Autodesk Fusion 360 part; units mm, degrees
sketch "Sketch1" plane through (0, 0, 0) normal (1, 0, 0) x (0, 0, -1)
  circle A0 centre (0, 0) radius 4
  line L0 (2, 2) -> (-2, 2)
  line L1 (-2, 2) -> (-2, -2)
  line L2 (-2, -2) -> (2, -2)
  line L3 (2, -2) -> (2, 2)
  line L4 (2, 2) -> (-2, -2) construction
  line L5 (-2, 2) -> (2, -2) construction
  dimension "d1" = 8
  dimension "d2" = 4
  dimension "d3" = 4
extrude "Extrude1" add sketch "Sketch1" along normal blind 2
sketch "Sketch2" plane through (2, 0, 0) normal (1, 0, 0) x (0, 0, -1)
  line L0 (2, 2) -> (2, -2)
  line L1 (2, -2) -> (-2, -2)
  line L2 (-2, -2) -> (-2, 2)
  line L3 (-2, 2) -> (2, 2)
  circle A0 centre (0, 0) radius 4
  circle A1 centre (0, 0) radius 7.5
  dimension "d6" = 15
extrude "Extrude2" add sketch "Sketch2" along normal blind 2 contours L0 L1 L2 L3 | A0 | A1
fillet "Fillet1" radius 1 1 edges at (2, -1.4465, 3.7293)
chamfer "Chamfer1" distance 0.5 angle 45 1 edges at (4, -2.7121, 6.9925)
sketch "Sketch3" plane through (4, 0, 0) normal (1, 0, 0) x (0, 0, -1)
  circle A0 centre (0, 0) radius 7
  line L0 (0, 0) -> (0, 2)
  line L1 (0, -4.8) -> (2, -4.8)
  line L2 (2, -4.8) -> (2, -5.6)
  line L3 (2, -5.6) -> (-2, -5.6)
  line L4 (-2, -5.6) -> (-2, -4.8)
  line L5 (0, -4.8) -> (-2, -4.8)
  line L6 (0, -3) -> (1.5, -3)
  line L7 (0, -3.8) -> (1.5, -3.8)
  line L8 (0, -3) -> (-1.5, -3)
  line L9 (0, -3.8) -> (-1.5, -3.8)
  line L10 (2.5, 2) -> (2.5, 0)
  line L11 (-2.5, 2) -> (-2.5, 0)
  line L12 (-1.7, 2) -> (-2.5, 2) construction
  line L13 (0, 2) -> (2.5, 2) construction
  line L14 (-1.7, 2) -> (-1.7, 0)
  line L15 (1.7, 2) -> (1.7, 0)
  arc A1 (-1.6925, 0.16) -> (1.6925, 0.16) centre (0, 0) ccw
  arc A2 (1.6925, 1.84) -> (-1.6925, 1.84) centre (0, 2) ccw
  arc A3 (-1.6925, 1.84) -> (-1.7, 1.833) centre (0, 0) ccw
  arc A4 (-1.7, 0.167) -> (-1.6925, 0.16) centre (0, 2) ccw
  arc A5 (-2.5, 0) -> (2.5, 0) centre (0, 0) ccw
  arc A6 (1.7, 1.833) -> (1.6925, 1.84) centre (0, 0) ccw
  arc A7 (1.6925, 0.16) -> (1.7, 0.167) centre (0, 2) ccw
  arc A8 (2.5, 2) -> (-2.5, 2) centre (0, 2) ccw
  line L16 (3, -1.5) -> (3.8, -1.5)
  arc A9 (1.5, -3) -> (3, -1.5) centre (1.5, -1.5) ccw
  arc A10 (1.5, -3.8) -> (3.8, -1.5) centre (1.5, -1.5) ccw
  line L17 (-3, -1.5) -> (-3.8, -1.5)
  arc A11 (-3.8, -1.5) -> (-1.5, -3.8) centre (-1.5, -1.5) ccw
  arc A12 (-3, -1.5) -> (-1.5, -3) centre (-1.5, -1.5) ccw
  line L18 (-0.4, -3.8) -> (0.4, -3.8)
  line L19 (0.4, -3.8) -> (0.4, -4.8)
  line L20 (0.4, -4.8) -> (-0.4, -4.8)
  line L21 (-0.4, -4.8) -> (-0.4, -3.8)
  dimension "d12" = 0.8
  dimension "d13" = 0.8
  dimension "d14" = 0.8
  dimension "d15" = 5
  dimension "d16" = 5
  dimension "d17" = 2
  dimension "d18" = 0.8
  dimension "d19" = 3
  dimension "d20" = 1.5
  dimension "d21" = 1.5
  dimension "d24" = 1.5
  dimension "d25" = 0.8
  dimension "d26" = 1.5
  dimension "d27" = 0.8
  dimension "d28" = 0.8
  dimension "d29" = 1.5
  dimension "d30" = 4
  dimension "d31" = 2
  dimension "d32" = 1
  dimension "d33" = 0.8
  dimension "d34" = 0.4
extrude "Extrude3" cut sketch "Sketch3" against normal blind 0.4 contours L1 L5 L7 L9 L18 L19 L20 L21 | L1 L2 L3 L4 L5 L20 | L6 L7 L8 L9 L16 A9 A10 L17 A11 A12 L18 | L10 L11 A5 A8
fillet "Fillet2" radius 0.4 12 edges at (3.8, -5.6, 2) (3.8, -4.8, 2) (3.8, -4.8, 0.4) (3.8, -3.8, 0.4) (3.8, -4.8, -2) (3.8, -5.6, -2) (3.8, -4.8, -0.4) (3.8, -3.8, -0.4) (3.8, -1.5, 3) (3.8, -1.5, 3.8) (3.8, -1.5, -3.8) (3.8, -1.5, -3)
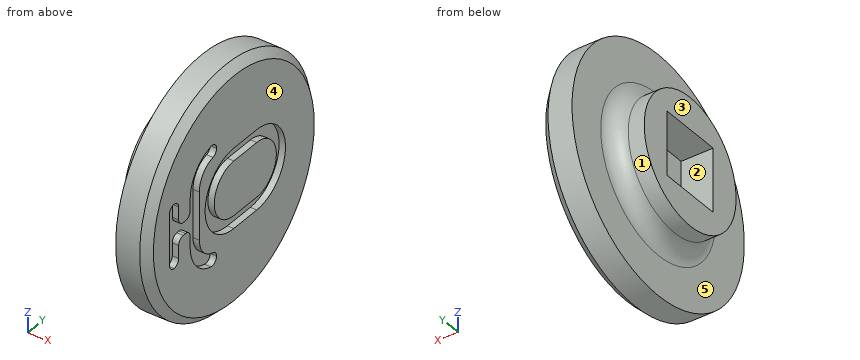
Verification items for the finished model (mm, model axes). Face numbers are marked on the shaded views. A direction names the side the tool comes from. Give positions to 0.01 mm unless a question says otherwise; leave off trailing zeros. Loops run counter-clockwise (first coordinate to the right, second up) from the corner with the lowest first, then second, coordinate; pieces in that order, holes last. Notation, with made-up numbers: (22, 31.5) - (26, 31.5) arc R22 ccw to (26, 69.5) - close; hole circle Ø8 at (69, 66). An arc over 180 degrees is marked (long way). Write item = value, one per line. Start each with the question number.
Q1. Tool access check on the marked faces 4 and 5. Record the directions out of +Z, -Z, +X, -X, +Y, -Y that give a thin tool (end or side, any length) a straight path to the whole face; none if there is none.
Q2. Cross-section at B-B, the plane x = 1.5. Enter the section's corners in (y, z).
Q3. Cross-section at A-A, the plane z = 0. Enter the section's corners in (x, y), and give its area (3 significant figures).
Q4. Thickness scan on line 1 (Y direction, x = 0.9, z = 0); line 2 (X direction, y = -3.25, z = 3.75); line 3 (Z direction, x = 3.8, y = 4.25). Record the ranges inside material, lowest first.
Q5. Mould release check, pull along Y, two halves, no side actions. Record for the marked faces 1, 2 and 3: released by +Y, released by -Y, zero draft, split by the parting line, or undercut.
Q6. Depth check by flat-ended pin: P1, Ø2, axis at y = 5.5, z = 3, coming from the -X side; P2, Ø3, axis at y = -3.5, z = -4.5, coming from the -X side. Enter the tip coordinate at first touch or a pass-through.
Answer key:
q1.face_4 = +Z, -Z, +X, +Y, -Y
q1.face_5 = -X
q2.outline = circle Ø8.27 at (0, 0); hole (-2, -2) - (2, -2) - (2, 2) - (-2, 2) - close
q3.outline = (0, -4) - (1, -4) arc R1 cw to (2, -5) - (2, -7.5) - (3.5, -7.5) - (4, -7) - (4, -5.6) - (3.6, -5.6) - (3.6, -3) - (4, -3) - (4, -2.5) - (3.6, -2.5) - (3.6, -1.7) - (4, -1.7) - (4, 3.7) - (3.6, 3.7) - (3.6, 4.5) - (4, 4.5) - (4, 7) - (3.5, 7.5) - (2, 7.5) - (2, 5) arc R1 cw to (1, 4) - (0, 4) - (0, 2) - (2, 2) - (2, -2) - (0, -2) - close
q3.area = 36.5 mm^2
q4.line_1 = -4 to -2, 2 to 4
q4.line_2 = 2 to 4
q4.line_3 = -5.81 to -1.09, 1.09 to 5.81
q5.face_1 = split by the parting line
q5.face_2 = undercut
q5.face_3 = zero draft
q6.P1 = 2
q6.P2 = 1.6
